Job drawing, mm, ordinate dimensions from the low corner. One solid piece. A direction names the side the tool comes from. Round coordinates to 2 decimals unless told otherwise and drop trailing zeros. Loops run counter-clockwise (first coordinate to the right, second up) from the corner with the lowest first, then second, coordinate; pieces in that order, holes last. Notation, with made-up numbers: M -39.5,59.25 L -21.5,59.25 A19 cw -21.5,91.25 Z; hole C 84,0 d1. An arc over 180 degrees is marked long. One line per item, written item: value.
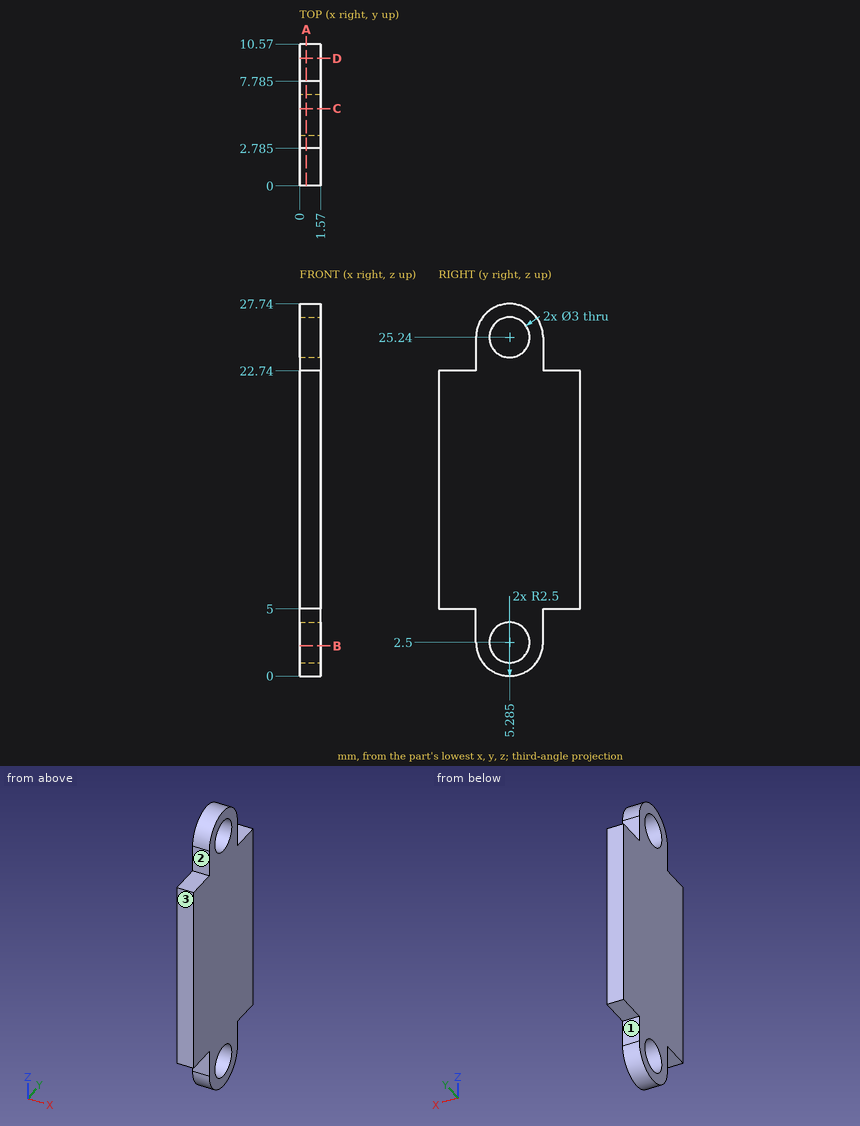
Item 1: Slice it at A-A, the plane x = 0.5. Give the cut face in (y, z) (3 decimals), and give its area (3 significant figures).
Check values:
outline: M 0,5 L 2.785,5 L 2.785,2.5 A2.5 ccw 7.785,2.5 L 7.785,5 L 10.57,5 L 10.57,22.74 L 7.785,22.74 L 7.785,25.24 A2.5 ccw 2.785,25.24 L 2.785,22.74 L 0,22.74 Z; hole C 5.285,2.5 d3; hole C 5.285,25.24 d3
area: 218 mm2
Item 2: Slice it at C-C, the plane y = 5.75. Give the cut face in (x, z), and give its area (3 significant figures).
Check values:
outline: M 0,0.04 L 1.57,0.04 L 1.57,1.07 L 0,1.07 Z; M 0,3.93 L 1.57,3.93 L 1.57,23.81 L 0,23.81 Z; M 0,26.67 L 1.57,26.67 L 1.57,27.7 L 0,27.7 Z
area: 34.5 mm2
Item 3: Wall check: line 1 along Z through (x, y) = (0.6, 5); line 2 along Y through (x, z) = (0.75, 23) (3 decimals); line 3 along Z through (x, y) = (1.45, 8.5). Give the ranges that are in metal, low to high.
Check values:
line 1: z = 0.02 to 1.03, 3.97 to 23.77, 26.71 to 27.72
line 2: y = 2.785 to 7.785
line 3: z = 5 to 22.74
Item 4: Drop flat-ended pins along their axis: P1, Ø0.5, axis at x = 0.5, z = 3.5, coming from the +Y side (3 decimals); P2, Ø2.5, axis at y = 5.285, z = 25.24, coming from the -X side; P3, Ø0.5, axis at x = 0.5, y = 9, coming from the +Z side; P4, Ø0.8, axis at x = 0.5, z = 23.5, coming from the -Y side (3 decimals). Give the stop position or say it passes through.
Check values:
P1: stops at y = 7.785
P2: passes through
P3: stops at z = 22.74
P4: stops at y = 2.785
Item 5: Slice it at B-B, the plane z = 2.25. Give the cut face in (x, y).
Check values:
outline: M 0,2.8 L 1.57,2.8 L 1.57,3.81 L 0,3.81 Z; M 0,6.76 L 1.57,6.76 L 1.57,7.77 L 0,7.77 Z
Item 6: Slice it at D-D, the plane y = 9.5. Give the cut face in (x, z), and give its area (3 significant figures).
Check values:
outline: M 0,5 L 1.57,5 L 1.57,22.74 L 0,22.74 Z
area: 27.9 mm2
Item 7: Which spindle directions (+Z, -Z, +X, -X, +Y, -Y) get a long thin tool onto all of the face, cutting with end or side? Do the marked faces 1, 2 and 3. Say none if no direction does.
Check values:
face 1: -Z, +X, -X, +Y
face 2: +Z, +X, -X, -Y
face 3: +Z, -Z, +X, -X, -Y
